Geometry check sheet. Reference: the model listing, model coordinates, mm. A direction names the side the tool comes from. Coordinates: 2 decimals unless noted, no trailing zeros. Write each loop counter-clockwise with the first axis right and the second up, starting at its lowest first coordinate (ties: lowest second). Pieces come first, ordered by that corner, then holes. Notation, with made-up numbers: M 88.5,-5.75 L 130.5,-5.75 A21 ccw 130.5,4.25 Z; hole C -36,85 d3. An arc over 180 degrees is marked long. Answer as a JSON object with one key per item and string values. Group by question number.
```python
from build123d import *

# Parameters (mm, degrees)
SKETCH1_W               = 10.16
SKETCH1_H               = 9.652
BOSS_EXTRUDE1_DEPTH     = 7.112
CUT_EXTRUDE1_DEPTH      = 14.021061708
CUT_EXTRUDE1_DEPTH_BACK = 14.021061708
SKETCH2_R               = 1.5875
SKETCH7_W               = 10.16
SKETCH7_H               = 9.652
BOSS_EXTRUDE3_DEPTH     = 1.27
FILLET1_R               = 0.635
FILLET3_R               = 0.635
FILLET4_R               = 0.381
CUT_EXTRUDE3_DEPTH      = 14.485940976
CUT_EXTRUDE3_DEPTH_BACK = 14.485940976
FILLET9_R               = 0.254
CUT_EXTRUDE7_DEPTH      = 9.654656319
SKETCH14_W              = 3.81
SKETCH14_H              = 3.302
BOSS_EXTRUDE4_DEPTH     = 10.16
FILLET14_R              = 1.27
FILLET15_R              = 0.254


with BuildPart() as part:
    # Sketch1 → Boss-Extrude1 (new body)
    with BuildSketch(Plane.XY):
        Rectangle(SKETCH1_W, SKETCH1_H)
        Polygon((-4.318, -3.81), (4.318, -3.81), (4.318, -1.016), (3.302, -1.016), (3.302, 2.794), (-3.302, 2.794), (-3.302, -1.016), (-4.318, -1.016), align=None, mode=Mode.SUBTRACT)
    extrude(amount=BOSS_EXTRUDE1_DEPTH)

    # Sketch2 → Cut-Extrude1 (cut, two sides: drawn at the far end of the back side and taken through both)
    with BuildSketch(Plane(origin=(0, 4.826, 0), x_dir=(1, 0, 0), z_dir=(0, 1, 0)).offset(-CUT_EXTRUDE1_DEPTH_BACK)):
        with Locations(Location((0, -2.794, 0), (0, 0, 90))):
            Circle(SKETCH2_R)
    extrude(amount=CUT_EXTRUDE1_DEPTH + CUT_EXTRUDE1_DEPTH_BACK, mode=Mode.SUBTRACT)

    # Sketch7 → Boss-Extrude3 (add)
    with BuildSketch(Plane.XY.offset(7.112)):
        Rectangle(SKETCH7_W, SKETCH7_H)
    extrude(amount=BOSS_EXTRUDE3_DEPTH)

    # Fillet1
    fillet1_edges = [part.edges().sort_by_distance(p)[0] for p in [
        (-5.08, 0, 0),
        (0, 4.826, 0),
        (5.08, 0, 0),
    ]]
    fillet(fillet1_edges, radius=FILLET1_R)

    # Fillet3
    # the kernel refuses this fillet: 0.635 mm, written as the material it takes off along each edge
    with BuildSketch(Plane(origin=(4.445, 4.191, 0.635), x_dir=(1, 0, 0), z_dir=(0, 1, 0))) as fillet3_piece_1_section:
        Polygon((0, 0), (FILLET3_R, 0), (FILLET3_R, FILLET3_R), (0, FILLET3_R), align=None)
    fillet3_piece_1 = extrude(amount=FILLET3_R, mode=Mode.PRIVATE)
    fillet3_piece_1 = fillet3_piece_1 - Plane(origin=(4.445, 4.191, 0.635), x_dir=(-0.7071067811865475, 0, 0.7071067811865475), z_dir=(0, 1, 0)) * Sphere(FILLET3_R, mode=Mode.PRIVATE)
    add(fillet3_piece_1, mode=Mode.SUBTRACT)
    with BuildSketch(Plane(origin=(-4.445, 4.191, 0.635), x_dir=(-1, 0, 0), z_dir=(0, 1, 0))) as fillet3_piece_2_section:
        Polygon((0, 0), (FILLET3_R, 0), (FILLET3_R, -FILLET3_R), (0, -FILLET3_R), align=None)
    fillet3_piece_2 = extrude(amount=FILLET3_R, mode=Mode.PRIVATE)
    fillet3_piece_2 = fillet3_piece_2 - Plane(origin=(-4.445, 4.191, 0.635), x_dir=(0.7071067811865475, 0, 0.7071067811865475), z_dir=(0, 1, 0)) * Sphere(FILLET3_R, mode=Mode.PRIVATE)
    add(fillet3_piece_2, mode=Mode.SUBTRACT)
    with BuildSketch(Plane(origin=(-4.445, -4.191, 7.747), x_dir=(0, 0, 1), z_dir=(-1, 0, 0))) as fillet3_piece_3_section:
        Polygon((0, 0), (FILLET3_R, 0), (FILLET3_R, -FILLET3_R), (0, -FILLET3_R), align=None)
    fillet3_piece_3 = extrude(amount=FILLET3_R, mode=Mode.PRIVATE)
    fillet3_piece_3 = fillet3_piece_3 - Plane(origin=(-4.445, -4.191, 7.747), x_dir=(0, 0.7071067811865475, -0.7071067811865475), z_dir=(-1, 0, 0)) * Sphere(FILLET3_R, mode=Mode.PRIVATE)
    add(fillet3_piece_3, mode=Mode.SUBTRACT)
    with BuildSketch(Plane(origin=(-4.445, 4.191, 7.747), x_dir=(-1, 0, 0), z_dir=(0, 1, 0))) as fillet3_piece_4_section:
        Polygon((0, 0), (FILLET3_R, 0), (FILLET3_R, FILLET3_R), (0, FILLET3_R), align=None)
    fillet3_piece_4 = extrude(amount=FILLET3_R, mode=Mode.PRIVATE)
    fillet3_piece_4 = fillet3_piece_4 - Plane(origin=(-4.445, 4.191, 7.747), x_dir=(0.7071067811865475, 0, -0.7071067811865475), z_dir=(0, 1, 0)) * Sphere(FILLET3_R, mode=Mode.PRIVATE)
    add(fillet3_piece_4, mode=Mode.SUBTRACT)
    with BuildSketch(Plane(origin=(4.445, -4.191, 7.747), x_dir=(1, 0, 0), z_dir=(0, 0, 1))) as fillet3_piece_5_section:
        Polygon((0, 0), (FILLET3_R, 0), (FILLET3_R, -FILLET3_R), (0, -FILLET3_R), align=None)
    fillet3_piece_5 = extrude(amount=FILLET3_R, mode=Mode.PRIVATE)
    fillet3_piece_5 = fillet3_piece_5 - Plane(origin=(4.445, -4.191, 7.747), x_dir=(-0.7071067811865476, 0.7071067811865475, 0), z_dir=(0, 0, 1)) * Sphere(FILLET3_R, mode=Mode.PRIVATE)
    add(fillet3_piece_5, mode=Mode.SUBTRACT)
    with BuildSketch(Plane(origin=(4.445, 4.191, 7.747), x_dir=(0, 0, 1), z_dir=(0, 1, 0))) as fillet3_piece_6_section:
        Polygon((0, 0), (FILLET3_R, 0), (FILLET3_R, FILLET3_R), (0, FILLET3_R), align=None)
    fillet3_piece_6 = extrude(amount=FILLET3_R, mode=Mode.PRIVATE)
    fillet3_piece_6 = fillet3_piece_6 - Plane(origin=(4.445, 4.191, 7.747), x_dir=(-0.7071067811865475, 0, -0.7071067811865475), z_dir=(0, 1, 0)) * Sphere(FILLET3_R, mode=Mode.PRIVATE)
    add(fillet3_piece_6, mode=Mode.SUBTRACT)
    with BuildSketch(Plane(origin=(-5.08, -4.191, 8.382), x_dir=(0, 0, -1), z_dir=(0, 1, 0))) as fillet3_piece_7:
        with BuildLine():
            CenterArc((FILLET3_R, -FILLET3_R), FILLET3_R, 90, 90)
            Line((0, -FILLET3_R), (0, 0))
            Line((0, 0), (FILLET3_R, 0))
        make_face()
    extrude(amount=8.382, mode=Mode.SUBTRACT)
    with BuildSketch(Plane(origin=(4.445, -4.826, 8.382), x_dir=(0, 1, 0), z_dir=(-1, 0, 0)), Plane(origin=(4.445, -4.826, 0), x_dir=(0, 0, 1), z_dir=(-1, 0, 0))) as fillet3_piece_8:
        with BuildLine():
            CenterArc((FILLET3_R, FILLET3_R), FILLET3_R, 180, 90)
            Line((0, FILLET3_R), (0, 0))
            Line((0, 0), (FILLET3_R, 0))
        make_face()
    extrude(amount=8.89, mode=Mode.SUBTRACT)
    with BuildSketch(Plane(origin=(5.08, 4.191, 8.382), x_dir=(-1, 0, 0), z_dir=(0, -1, 0))) as fillet3_piece_9:
        with BuildLine():
            CenterArc((FILLET3_R, FILLET3_R), FILLET3_R, 180, 90)
            Line((0, FILLET3_R), (0, 0))
            Line((0, 0), (FILLET3_R, 0))
        make_face()
    extrude(amount=8.382, mode=Mode.SUBTRACT)
    with BuildSketch(Plane(origin=(-4.445, 4.826, 8.382), x_dir=(0, 0, -1), z_dir=(1, 0, 0))) as fillet3_piece_10:
        with BuildLine():
            CenterArc((FILLET3_R, -FILLET3_R), FILLET3_R, 90, 90)
            Line((0, -FILLET3_R), (0, 0))
            Line((0, 0), (FILLET3_R, 0))
        make_face()
    extrude(amount=8.89, mode=Mode.SUBTRACT)
    with BuildSketch(Plane(origin=(4.445, -4.826, 0.635), x_dir=(0, 0, -1), z_dir=(-1, 0, 0))) as fillet3_piece_11:
        with BuildLine():
            CenterArc((0.635 - FILLET3_R, -FILLET3_R), FILLET3_R, 0, 90)
            Line((0.635, -FILLET3_R), (0.635, 0))
            Line((0.635, 0), (0.635 - FILLET3_R, 0))
        make_face()
    revolve(axis=Axis((4.445, -4.826, 0.635), (0, -1, 0)), revolution_arc=90, mode=Mode.SUBTRACT)
    with BuildSketch(Plane(origin=(-4.445, -4.826, 0.635), x_dir=(0, 0, -1), z_dir=(1, 0, 0))) as fillet3_piece_12:
        with BuildLine():
            CenterArc((0.635 - FILLET3_R, FILLET3_R), FILLET3_R, 270, 90)
            Line((0.635, FILLET3_R), (0.635, 0))
            Line((0.635, 0), (0.635 - FILLET3_R, 0))
        make_face()
    revolve(axis=Axis((-4.445, -4.826, 0.635), (0, 1, 0)), revolution_arc=90, mode=Mode.SUBTRACT)
    with BuildSketch(Plane(origin=(5.08, -4.826, 7.747), x_dir=(0, 1, 0), z_dir=(0, 0, -1)), Plane(origin=(-5.08, -4.826, 0.635), x_dir=(0, 1, 0), z_dir=(0, 0, 1)), Plane(origin=(-5.08, 4.826, 0.635), x_dir=(1, 0, 0), z_dir=(0, 0, 1)), Plane(origin=(5.08, 4.826, 7.747), x_dir=(-1, 0, 0), z_dir=(0, 0, -1))) as fillet3_piece_13:
        with BuildLine():
            CenterArc((FILLET3_R, -FILLET3_R), FILLET3_R, 90, 90)
            Line((0, -FILLET3_R), (0, 0))
            Line((0, 0), (FILLET3_R, 0))
        make_face()
    extrude(amount=7.112, mode=Mode.SUBTRACT)

    # Fillet4
    fillet4_edges = [part.edges().sort_by_distance(p)[0] for p in [
        (3.302, -1.016, 3.556),
        (-3.302, -1.016, 3.556),
    ]]
    fillet(fillet4_edges, radius=FILLET4_R)

    # Sketch11 → Cut-Extrude3 (cut, two sides: drawn at the far end of the back side and taken through both)
    with BuildSketch(Plane.ZY.offset(-4.318).offset(-CUT_EXTRUDE3_DEPTH_BACK)):
        Polygon((0, -3.81), (5.08, -3.81), (5.08, -4.064), (10.16, -4.826), (0, -4.826), align=None)
    extrude(amount=CUT_EXTRUDE3_DEPTH + CUT_EXTRUDE3_DEPTH_BACK, mode=Mode.SUBTRACT)

    # Fillet9
    fillet9_edges = [part.edges().sort_by_distance(p)[0] for p in [
        (-4.318, -3.81, 6.096),
        (4.318, -3.81, 6.096),
        (0, -3.81, 7.112),
    ]]
    fillet(fillet9_edges, radius=FILLET9_R)

    # Sketch13 → Cut-Extrude7 (cut, through all)
    with BuildSketch(Plane(origin=(0, 0, 5.08), x_dir=(-1, 0, 0), z_dir=(0, 0, -1))):
        Polygon((-5.08, -3.81), (-5.08, -4.826), (-2.032, -4.826), align=None)
        Polygon((5.08, -3.81), (5.08, -4.826), (2.032, -4.826), align=None)
    extrude(amount=-CUT_EXTRUDE7_DEPTH, mode=Mode.SUBTRACT)

    # Sketch14 → Boss-Extrude4 (add)
    with BuildSketch(Plane.XY.offset(8.382)):
        Rectangle(SKETCH14_W, SKETCH14_H)
    extrude(amount=BOSS_EXTRUDE4_DEPTH)

    # Fillet14
    fillet14_edges = [part.edges().sort_by_distance(p)[0] for p in [
        (0, 1.651, 8.382),
        (-1.905, 0, 8.382),
        (0, -1.651, 8.382),
        (1.905, 0, 8.382),
    ]]
    fillet(fillet14_edges, radius=FILLET14_R)

    # Fillet15
    fillet15_edges = [part.edges().sort_by_distance(p)[0] for p in [
        (1.905, 1.651, 14.097),
        (-1.905, 1.651, 14.097),
        (-1.905, -1.651, 14.097),
        (1.905, -1.651, 14.097),
        (0, 1.651, 18.542),
        (-1.905, 0, 18.542),
        (0, -1.651, 18.542),
        (1.905, 0, 18.542),
        (2.354517888, 2.100517888, 8.682614059),
        (2.354517888, -2.100517888, 8.682614059),
        (-2.354517888, 2.100517888, 8.682614059),
        (-2.354517888, -2.100517888, 8.682614059),
    ]]
    fillet(fillet15_edges, radius=FILLET15_R)


solid = part.part
```
1) Go/stop test with flat-tipped pins: pin 1 Ø1.5 at (x, y) = (1.5, 0.5) entering from -Z; pin 2 Ø0.6 at (x, z) = (4.5, 1.5) entering from -Y; pin 3 Ø3.5 at (x, z) = (0.5, 2.5) entering from -Y. Record where each tip stops, or that it passes through.
2) Set-up check for faces 4 (the flat face through (1.905, 0, 14)), 5 (the flat face through (0, 2.794, 5)), 6 (the flat face through (-1.905, 0, 14)): record each of +Z, -Z, +X, -X, +Y, -Y from which the full face is reachable in a straight line by a thin tool's end or side.
3) Draft check along Z on faces 1 (the flat face through (4.318, -2, 4)), 2 (the cylindrical face through (-0.07, 3.8, 4.38)), 3 (the cylindrical face through (0.044, -2.204, 8.604)). Enter one of: +Z half, -Z half, draft (parallel to the pull), parting line (faces both ways), or undercut.
4) Section check D-D (z = 11.25). Record the cut outline in (x, y) (3 decimals), then the cut area to 3 significant figures.
5) Section check C-C (y = -3.25). Record the cut outline in (x, z) (3 decimals).
6) Section check B-B (z = 1.5). Record the cut outline in (x, y) (3 decimals).
7) Material ranges on probe 1 along X at (y, z) = (2.75, 1); probe 2 along Y at (x, z) = (1.5, 10.25); probe 3 along Z at (x, y) = (-3.25, -2.5), recorded low to high. Write a range as [from, to].
Entries:
{
 "1": {"pin 1": "z = 7.11", "pin 2": "y = -3.81", "pin 3": "y = 2.79"},
 "2": {"face 4": "+Z, +X, +Y, -Y", "face 5": "-Z", "face 6": "+Z, -X, +Y, -Y"},
 "3": {"face 1": "draft", "face 2": "undercut", "face 3": "+Z half"},
 "4": {"outline": "M -1.905,-1.397 A0.254 ccw -1.651,-1.651 L 1.651,-1.651 A0.254 ccw 1.905,-1.397 L 1.905,1.397 A0.254 ccw 1.651,1.651 L -1.651,1.651 A0.254 ccw -1.905,1.397 Z", "area": "12.5 mm^2"},
 "5": {"outline": "M -5.08,0.635 A0.635 ccw -4.445,0 L -4.318,0 L -4.318,7.112 L 4.318,7.112 L 4.318,0 L 4.445,0 A0.635 ccw 5.08,0.635 L 5.08,7.747 A0.635 ccw 4.445,8.382 L -4.445,8.382 A0.635 ccw -5.08,7.747 Z"},
 "6": {"outline": "M -5.08,-3.81 L -4.318,-3.81 L -4.318,-1.016 L -3.683,-1.016 A0.381 ccw -3.302,-0.635 L -3.302,2.794 L -0.92,2.794 L -0.92,4.826 L -4.445,4.826 A0.635 ccw -5.08,4.191 Z; M 0.92,2.794 L 3.302,2.794 L 3.302,-0.635 A0.381 ccw 3.683,-1.016 L 4.318,-1.016 L 4.318,-3.81 L 5.08,-3.81 L 5.08,4.191 A0.635 ccw 4.445,4.826 L 0.92,4.826 Z"},
 "7": {"probe 1": "[-5.08, -3.3], [3.3, 5.08]", "probe 2": "[-1.65, 1.65]", "probe 3": "[7.11, 8.38]"}
}
